For this review, use the dimensioned drawing (mm, ordinates from the lowest corner) and the shaded views. A direction names the side the tool comes from. Give positions to 0.01 mm unless a question says otherwise; leave off trailing zeros. Order: outer loops, then holes, each group sorted by start corner. A loop starts at its lowest first (then second) coordinate and runs counter-clockwise, first axis right, second up.
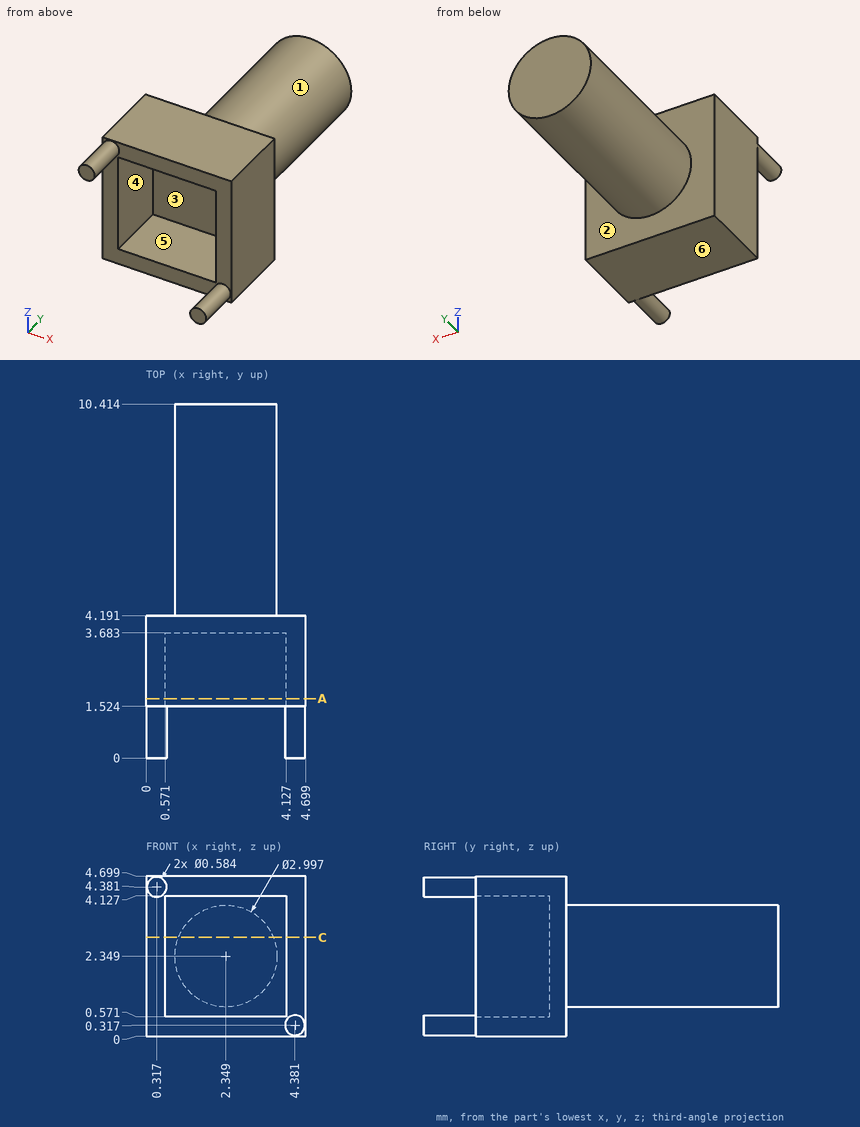
1. Take a section at C-C (z = 2.9). Write out the cut boundary in (x, y) (1 decimal).
2. Insertion check: pin 1 (1 mm diameter, centred on y = 5.5, z = 1.5, fed in from -X); pin 2 (1.8 mm diameter, centred on x = 2.5, z = 2.5, fed in from -Y). Each pin has a flat end and moves straight along its axis. Give the tip position at first contact, or say it passes through.
3. For the marked faces 5 and 6, list the 3-axis set-ups (+Z, -Z, +X, -X, +Y, -Y) from which the entire face can be reached by the end or side of a thin tool; tool diameter is ignored.
4. Take a section at A-A (y = 1.75). Write out the cut boundary in (x, z).
5. To check wall thickness, follow line 1 (Z direction, x = 3, y = 3.5); line 2 (Y direction, x = 4.4, z = 1.75) (1 decimal). State the ranges of each line that lie inside material, in increasing order.
6. Draft analysis for pull direction Z (two halves, no side actions). For the marked faces 1, 2, 3 and 4, state which applies: pulls with the +Z half, pulls with the -Z half, needs draft (parallel to the pull), parting line crosses it, or undercut.
Answer:
1. outline: (0, 1.5) - (0.6, 1.5) - (0.6, 3.7) - (4.1, 3.7) - (4.1, 1.5) - (4.7, 1.5) - (4.7, 4.2) - (3.7, 4.2) - (3.7, 10.4) - (1, 10.4) - (1, 4.2) - (0, 4.2) - close
2. pin 1: stops at x = 0.89
2. pin 2: stops at y = 3.68
3. face 5: -Y
3. face 6: -Z, +X, -X, +Y, -Y
4. outline: (0, 0) - (4.7, 0) - (4.7, 4.7) - (0, 4.7) - close; hole (0.57, 0.57) - (4.13, 0.57) - (4.13, 4.13) - (0.57, 4.13) - close
5. line 1: z = 0 to 0.57, 4.13 to 4.7
5. line 2: y = 1.5 to 4.2
6. face 1: parting line crosses it
6. face 2: needs draft
6. face 3: undercut
6. face 4: undercut
